The figure shows three views and two pictorial views of one solid part (mm, origin at its lowest corner). Answer the questions. Round coordinates to 2 decimals unless told otherwise and drop trailing zeros. Write each loop counter-clockwise with the first axis right and the second up, starting at its lowest first coordinate (ties: lowest second). Pieces come first, ordered by that corner, then holes.
Item 1: Find section A-A on y = 80. Give the vertices of the cut face in (x, z), then the cut area to 3 significant figures.
Item 2: This flat-tipped pin is pushed along its axis until it touches: pin 1 (1 mm diameter, centred on x = 0.5, y = 104, fed in from -Z). Where does it stop, or does it pass through?
Item 3: Find section C-C on y = 98. Give the vertices of the cut face in (x, z).
Item 4: Find section B-B on z = 30. Give the vertices of the cut face in (x, y).
Item 5: Find the intervals of material crossed by probe 1 along Z at (x, y) = (1.55, 80); probe 2 along Z at (x, y) = (1.3, 10); probe 3 along Z at (x, y) = (0.1, 96), in increasing order.
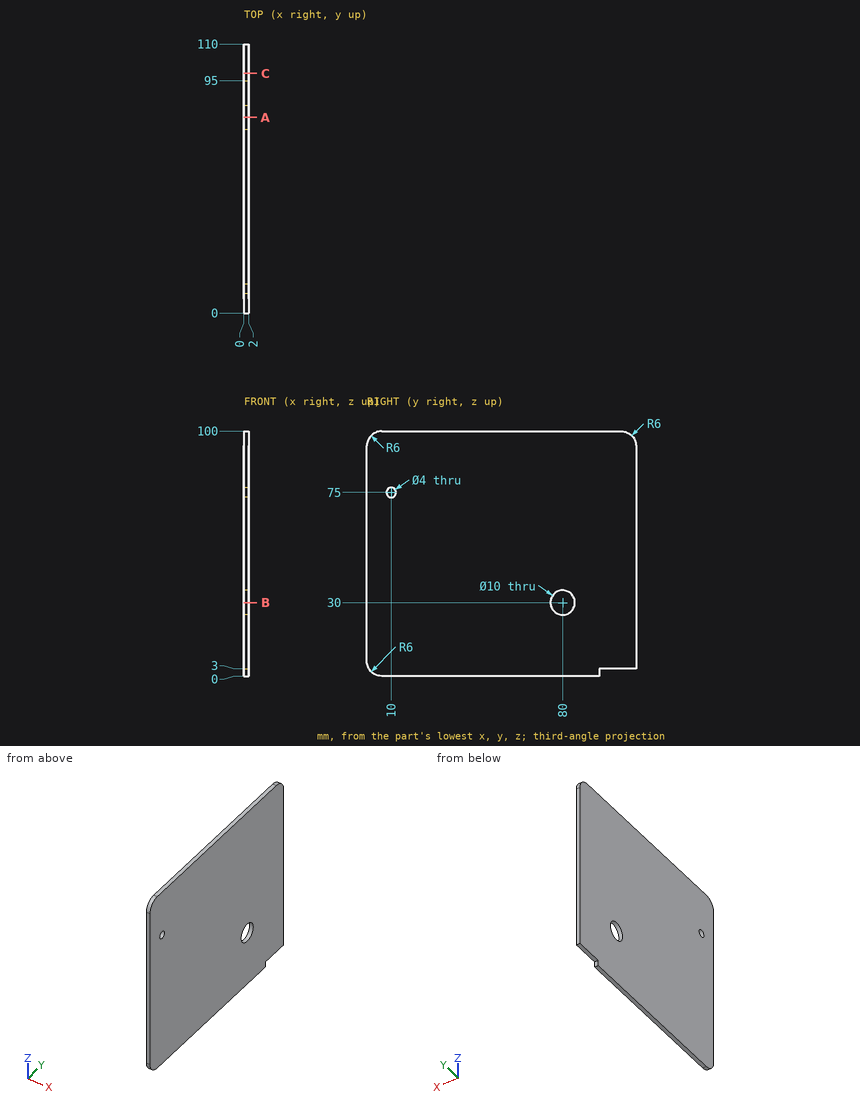
Check values:
1. outline: (0, 0) - (2, 0) - (2, 25) - (0, 25) - close; (0, 35) - (2, 35) - (2, 100) - (0, 100) - close
1. area: 180 mm2
2. pin 1: stops at z = 3
3. outline: (0, 3) - (2, 3) - (2, 100) - (0, 100) - close
4. outline: (0, 0) - (2, 0) - (2, 75) - (0, 75) - close; (0, 85) - (2, 85) - (2, 110) - (0, 110) - close
5. probe 1: z = 0 to 25, 35 to 100
5. probe 2: z = 0 to 73, 77 to 100
5. probe 3: z = 3 to 100
